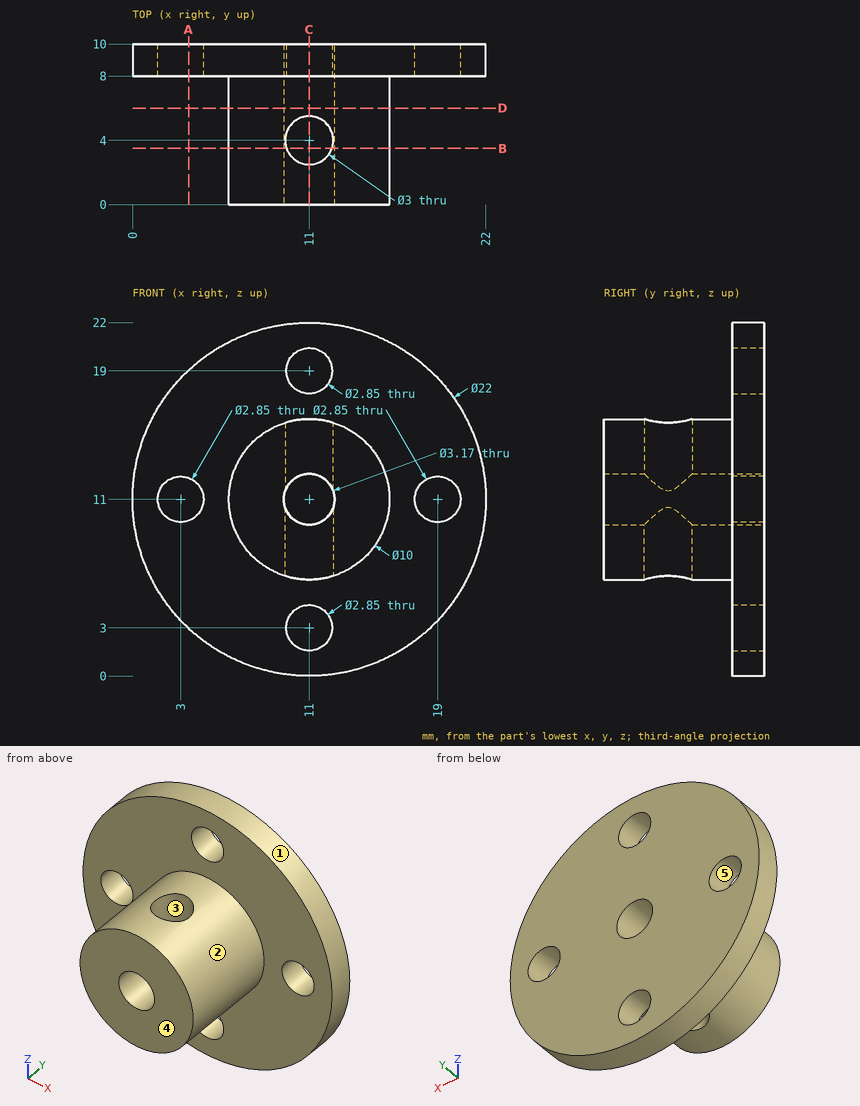
Study the drawing (mm; zero at the part's minimum x, y, z) and answer. A direction names the side the tool comes from. Give positions to 0.01 mm unless a question says otherwise; leave off trailing zeros. Order: outer loops, then holes, each group sorted by start corner. A loop starts at its lowest first (then second) coordinate and runs counter-clockwise, first axis right, second up. Notation, with made-up numbers: (76, 29.25) - (87, 29.25) arc R22 ccw to (87, 46.25) - close; hole circle Ø1 at (82, 24). An arc over 180 degrees is marked (long way). Answer as CSV lines item,"result". Start each with the question number.
Q1. The part is cut by section A-A (x = 3.5). Write down the section's boundary in (y, z).
Q2. The part is cut by section B-B (y = 3.5). Write down the section's boundary in (x, z) (3 decimals).
Q3. The mould has two halves that part along Y. Classify the marked faces 3, 4 and 5: +Y half, -Y half, draft (parallel to the pull), parting line (faces both ways), or undercut.
Q4. The part is cut by section C-C (x = 11). Write down the section's boundary in (y, z) (3 decimals).
Q5. Given pin 1 Ø3.5 at (x, z) = (19, 11) entering from -Y; pin 2 Ø2 at (x, y) = (6, 5) entering from -Z; pin 3 Ø2.5 at (x, z) = (11, 3) entering from -Y; pin 4 Ø1.5 at (y, z) = (8.5, 17) entering from +X, each flat-ended and moving along its own axis, determine where each tip first touches the part or whether it passes through.
Q6. Find the intervals of material crossed by L1, parallel to Z at x = 11, y = 9.4 (3 decimals); L2, parallel to Y at x = 11, z = 8.85, in increasing order. Write a range as [from, to].
Q7. The part is cut by section D-D (y = 6). Write down the section's boundary in (x, z) (3 decimals).
Q8. For the marked faces 1 and 2, determine the directions among +Z, -Z, +X, -X, +Y, -Y from which every point of the face is accessible in a straight line to the end or side of a thin tool.
Check result:
1,outline,"(8, 2.95) - (10, 2.95) - (10, 9.67) - (8, 9.67) - close; (8, 12.33) - (10, 12.33) - (10, 19.05) - (8, 19.05) - close"
2,outline,"(9.586, 6.204) - (9.586, 10.284) arc R1.585 cw to (9.586, 11.716) - (9.586, 15.796) arc R5 ccw to start; (12.414, 6.204) arc R5 ccw to (12.414, 15.796) - (12.414, 11.716) arc R1.585 cw to (12.414, 10.284) - close"
3,face 3,"undercut"
3,face 4,"-Y half"
3,face 5,"draft"
4,outline,"(0, 6) - (2.5, 6) - (2.5, 9.415) - (0, 9.415) - close; (0, 12.585) - (2.5, 12.585) - (2.5, 16) - (0, 16) - close; (5.5, 6) - (8, 6) - (8, 4.425) - (10, 4.425) - (10, 9.415) - (5.5, 9.415) - close; (5.5, 12.585) - (10, 12.585) - (10, 17.575) - (8, 17.575) - (8, 16) - (5.5, 16) - close; (8, 0) - (10, 0) - (10, 1.575) - (8, 1.575) - close; (8, 20.425) - (10, 20.425) - (10, 22) - (8, 22) - close"
5,pin 1,"stops at y = 8"
5,pin 2,"stops at z = 8"
5,pin 3,"passes through"
5,pin 4,"stops at x = 20.67"
6,L1,"z = [0, 1.575], [4.425, 9.415], [12.585, 17.575], [20.425, 22]"
6,L2,"y = [0, 2.5], [5.5, 10]"
7,outline,"circle Ø10 at (11, 11); hole circle Ø3.17 at (11, 11)"
8,face 1,"+Y, -Y"
8,face 2,"-Y"
